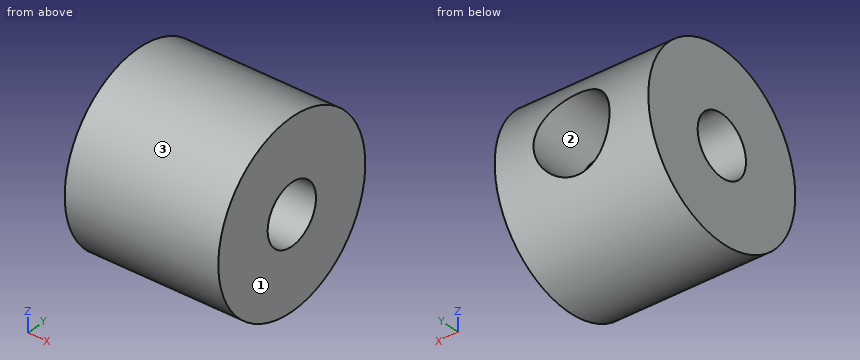
```python
from build123d import *

# Parameters (mm, degrees)
SCHIZZO1_R                        = 2.995
SCHIZZO1_R_2                      = 0.985
ESTRUSIONE_ESTRUSIONE1_DEPTH      = 5.05
FORO_FILETTATO_M3X0_5_1_OUTLINE_W = 1.25
FORO_FILETTATO_M3X0_5_1_OUTLINE_H = 2.995111585


# Read off the part's stored shape, not the designer's step: Foro filettato M3x0.5-1
with BuildPart() as part:
    # Schizzo1 → Estrusione-Estrusione1 (new body)
    with BuildSketch(Plane(origin=(0, 0, 0), x_dir=(0, 0, -1), z_dir=(1, 0, 0))):
        Circle(SCHIZZO1_R)
        Circle(SCHIZZO1_R_2, mode=Mode.SUBTRACT)
    extrude(amount=ESTRUSIONE_ESTRUSIONE1_DEPTH)

    # Foro filettato M3x0.5-1 outline → Foro filettato M3x0.5-1 (revolve, cut)
    with BuildSketch(Plane(origin=(2.525, 0, 0), x_dir=(1, 0, 0), z_dir=(0, 0, 1))):
        with Locations((0.625, 1.497555793)):
            Rectangle(FORO_FILETTATO_M3X0_5_1_OUTLINE_W, FORO_FILETTATO_M3X0_5_1_OUTLINE_H)
    revolve(axis=Axis((2.525, 0, 0), (0, 1, 0)), mode=Mode.SUBTRACT)


solid = part.part
```
Design review of the part built by this model. Coordinates are the model's own, in mm. Face numbers are marked on the shaded views. Coordinates: 2 decimals unless noted, no trailing zeros. Order: outer loops, then holes, each group sorted by start corner. A loop starts at its lowest first (then second) coordinate and runs counter-clockwise, first axis right, second up. Notation, with made-up numbers: (75, -10) -> (91, -10) arc R23 cw to (91, 26) -> close; hole circle Ø4 at (81, 72.25). An arc over 180 degrees is marked (long way). One line per item, written item: value. Start each with the question number.
Q1. Take a section at A-A, the plane z = 0. State the section outline as (x, y) points (3 decimals), then the cut area to 3 significant figures.
Q2. Take a section at C-C, the plane y = 1.8. State the section outline as (x, z) points (3 decimals), then the cut area to 3 significant figures.
Q3. Take a section at B-B, the plane y = -0.9. State the section outline as (x, z) points, then the cut area to 3 significant figures.
Q4. Take a section at D-D, the plane x = 0.8. State the section outline as (y, z) points (3 decimals), then the cut area to 3 significant figures.
Q5. Insertion check: pin 1 Ø2 at (x, z) = (2, -2) entering from -Y; pin 2 Ø3 at (x, z) = (3.5, 1.5) entering from -Y (3 decimals). Each pin has a flat end and moves straight along its axis. Give the tip position at first contact, or say it passes through.
Q6. For probe 1 along X at (y, z) = (2.45, 0) (3 decimals); probe 2 along Z at (x, y) = (4.6, -0.6); probe 3 along Z at (x, y) = (1.45, 1.1), list the stretches that pass through material, from the lowest coordinate up.
Q7. Mouldability with a two-part tool opening along Z and no side actions: class the marked faces 1, 2 and 3 as pulls with the +Z half, pulls with the -Z half, needs draft (parallel to the pull), parting line crosses it, or undercut.
Values follow:
1. outline: (0, -2.995) -> (5.05, -2.995) -> (5.05, -0.985) -> (0, -0.985) -> close; (0, 0.985) -> (1.275, 0.985) -> (1.275, 2.995) -> (0, 2.995) -> close; (3.775, 0.985) -> (5.05, 0.985) -> (5.05, 2.995) -> (3.775, 2.995) -> close
1. area: 15.3 mm2
2. outline: (0, -2.394) -> (5.05, -2.394) -> (5.05, 2.394) -> (0, 2.394) -> close; hole circle Ø2.5 at (2.525, 0)
2. area: 19.3 mm2
3. outline: (0, -2.86) -> (5.05, -2.86) -> (5.05, -0.4) -> (0, -0.4) -> close; (0, 0.4) -> (5.05, 0.4) -> (5.05, 2.86) -> (0, 2.86) -> close
3. area: 24.8 mm2
4. outline: circle Ø5.99 at (0, 0); hole circle Ø1.97 at (0, 0)
4. area: 25.1 mm2
5. pin 1: stops at y = -2.82
5. pin 2: stops at y = -2.995
6. probe 1: x = 0 to 1.275, 3.775 to 5.05
6. probe 2: z = -2.93 to -0.78, 0.78 to 2.93
6. probe 3: z = -2.79 to -0.64, 0.64 to 2.79
7. face 1: needs draft
7. face 2: undercut
7. face 3: parting line crosses it
